Check sheet for the modelled part. Datum: model origin and axes. Units: mm. Coordinates: 2 decimals unless noted, no trailing zeros. Order: outer loops, then holes, each group sorted by start corner. A loop starts at its lowest first (then second) coordinate and runs counter-clockwise, first axis right, second up.
1. Cross-section at C-C (z = -4). Enter the section's corners in (x, y), then the cut area to 3 significant figures.
2. Cross-section at D-D (z = 1.5). Enter the section's corners in (x, y).
3. Gauge pin test, flat ends, axial feed: pin 1 Ø8 at (x, y) = (-2.5, -2) entering from -Z; pin 2 Ø1.5 at (x, z) = (0.5, -1.5) entering from -Y; pin 3 Ø1.5 at (x, z) = (10, -4) entering from -Y; pin 4 Ø2 at (x, y) = (2, -3.5) entering from -Z. Record the tip position at first contact, or that the pin passes through.
4. Thickness scan on line 1 (Z direction, x = -7, y = -11); line 2 (Z direction, x = 2, y = -11.5); line 3 (Y direction, x = 0, z = -2.75). Record the ranges inside material, lowest first.
5. Cross-section at A-A (x = 0). Enter the section's corners in (y, z) (1 decimal), then the cut area to 3 significant figures.
Autodesk Inventor part; units mm, degrees
ref_plane "YZ Plane" through (0, 0, 0) normal (1, 0, 0) x (0, 1, 0)
ref_plane "XZ Plane" through (0, 0, 0) normal (0, 1, 0) x (-1, 0, 0)
ref_plane "XY Plane" through (0, 0, 0) normal (0, 0, 1) x (1, 0, 0)
sketch "Sketch1" plane through (0, 0, 0) normal (0, 1, 0) x (-1, 0, 0)
  line L0 (-6.4389, 0) -> (-6.4389, -7.167)
  line L1 (-14.605, -5.5) -> (-13.605, -4.3875)
  line L2 (-14.605, -7.167) -> (-14.605, -5.5)
  line L3 (-6.4389, -7.167) -> (-14.605, -7.167)
  line L4 (-6.4389, 0) -> (-6.4389, -7.167)
  arc A0 (-13.605, -4.3875) -> (-10.105, 0) centre (-14.605, 0) ccw
  line L5 (0, 7.167) -> (0, -7.167)
  line L6 (-10.105, 0) -> (-6.4389, 0)
  point P0 (0, 0)
  point P1 (0, 0)
  dimension "d0" = 12.8778
  dimension "d1" = 29.21
  dimension "d2" = 1.667
  dimension "d3" = 4.5
  dimension "d6" = 8.1661
  dimension "d7" = 1
  dimension "d8" = 11
revolve "Revolution1" add sketch "Sketch1" angle 360 about axis through (0, 0, 7.167) along (0, 0, -1)
mirror "Mirror1" about plane through (10.105, 0, 0) normal (0, 0, 1)
properties part number "TTB 4mm Dyneema Cable Pulley" material "Acetal Resin, Black"
Data:
1. outline: circle Ø25.09 at (0, 0); hole circle Ø12.88 at (0, 0)
1. area: 364 mm2
2. outline: circle Ø20.72 at (0, 0); hole circle Ø12.88 at (0, 0)
3. pin 1: stops at z = -7.17
3. pin 2: stops at y = -10.7
3. pin 3: stops at y = -9.96
3. pin 4: passes through
4. line 1: z = -7.17 to -4.22, 4.22 to 7.17
4. line 2: z = -7.17 to -3.41, 3.41 to 7.17
4. line 3: y = -11.04 to -6.44, 6.44 to 11.04
5. outline: (-14.6, -7.2) - (-6.4, -7.2) - (-6.4, 7.2) - (-14.6, 7.2) - (-14.6, 5.5) - (-13.6, 4.4) arc R4.5 cw to (-10.1, 0) arc R4.5 cw to (-13.6, -4.4) - (-14.6, -5.5) - close; (6.4, -7.2) - (14.6, -7.2) - (14.6, -5.5) - (13.6, -4.4) arc R4.5 cw to (10.1, 0) arc R4.5 cw to (13.6, 4.4) - (14.6, 5.5) - (14.6, 7.2) - (6.4, 7.2) - close
5. area: 169 mm2
